The model under review builds one solid part; all positions refer to its coordinate system, in mm. A direction names the side the tool comes from. Coordinates: 2 decimals unless noted, no trailing zeros. Loops run counter-clockwise (first coordinate to the right, second up) from the corner with the lowest first, then second, coordinate; pieces in that order, holes last. Notation, with made-up numbers: M 54,-18 L 75,-18 A19 ccw 75,12 Z; hole C -6,-16.5 d5. An arc over 180 degrees is marked long. One line per item, written item: value.
```python
from build123d import *

# Parameters (mm, degrees)
SKETCH1_W           = 192.5
SKETCH1_H           = 7.5
BOSS_EXTRUDE1_DEPTH = 92.5
SKETCH4_W           = 7.5
SKETCH4_H           = 7.5
CUT_EXTRUDE1_DEPTH  = 92.5


with BuildPart() as part:
    # Sketch1 → Boss-Extrude1 (new body)
    with BuildSketch(Plane(origin=(0, 0, 0), x_dir=(1, 0, 0), z_dir=(0, 1, 0))):
        with Locations((-96.25, 3.75)):
            Rectangle(SKETCH1_W, SKETCH1_H)
    extrude(amount=BOSS_EXTRUDE1_DEPTH)

    # Sketch4 → Cut-Extrude1 (cut)
    with BuildSketch(Plane.XY):
        with Locations((-3.75, 88.75)):
            Rectangle(SKETCH4_W, SKETCH4_H)
        with Locations((-3.75, 73.75)):
            Rectangle(SKETCH4_W, SKETCH4_H)
        with Locations((-3.75, 58.75)):
            Rectangle(SKETCH4_W, SKETCH4_H)
        with Locations((-3.75, 43.75)):
            Rectangle(SKETCH4_W, SKETCH4_H)
        with Locations((-3.75, 28.75)):
            Rectangle(SKETCH4_W, SKETCH4_H)
        with Locations((-3.75, 13.75)):
            Rectangle(SKETCH4_W, SKETCH4_H)
    extrude(amount=-CUT_EXTRUDE1_DEPTH, mode=Mode.SUBTRACT)


solid = part.part
```
(1) Tool access review of faces 1 (the face through (-4, 70, -4)), 2 (the face through (0, 66, -4)): name each direction out of +Z, -Z, +X, -X, +Y, -Y from which nothing blocks a thin tool from reaching the whole face with its end or side.
Checks:
face 1: +Z, -Z, +X
face 2: +Z, -Z, +X, +Y, -Y
(2) To check wall thickness, follow L1, parallel to X at y = 41, z = -5. State the ranges of the line that lie inside material, in increasing order. Write a range as [from, to].
Checks:
L1: [-192.5, -7.5]
(3) Draft analysis for pull direction Y (two halves, no side actions). For faces 3 (the face through (0, 51, -4)), 4 (the face through (-98, 0, -4)), 5 (the face through (-4, 25, -4)), 6 (the face through (-4, 85, -4)), state which applies: pulls with the +Y half, pulls with the -Y half, needs draft (parallel to the pull), parting line crosses it, or undercut.
Checks:
face 3: needs draft
face 4: pulls with the -Y half
face 5: undercut
face 6: pulls with the +Y half
(4) Add section A-A on z = -2.5. State the section outline as (x, y) points, then the cut area to 3 significant figures.
Checks:
outline: M -192.5,0 L 0,0 L 0,10 L -7.5,10 L -7.5,17.5 L 0,17.5 L 0,25 L -7.5,25 L -7.5,32.5 L 0,32.5 L 0,40 L -7.5,40 L -7.5,47.5 L 0,47.5 L 0,55 L -7.5,55 L -7.5,62.5 L 0,62.5 L 0,70 L -7.5,70 L -7.5,77.5 L 0,77.5 L 0,85 L -7.5,85 L -7.5,92.5 L -192.5,92.5 Z
area: 17,500 mm^2
(5) Insertion check: pin 1 Ø2 at (x, z) = (-5, -5.5) entering from +Y; pin 2 Ø2 at (x, z) = (-3.5, -3.5) entering from -Y; pin 3 Ø2 at (y, z) = (75.5, -5) entering from +X. Each pin has a flat end and moves straight along its axis. Give the tip position at first contact, or say it passes through.
Checks:
pin 1: y = 85
pin 2: y = 0
pin 3: x = -7.5
